from build123d import *

# Parameters (mm, degrees)
F0_R     = 6.604
F0_R_2   = 3.175
F1_DEPTH = 2.54
F2_R     = 10.414
F2_R_2   = 6.604
F2_R_3   = 3.175
F3_DEPTH = 3.81
F4_SIZE  = 3.80999
F6_DEPTH = 6.35


# Not quite as in the source:
# - a fillet or chamfer is up to 0.001 mm smaller than in the source, because OpenCascade refuses the exact size


with BuildPart() as f1:
    # F0 (on Top) → F1 (new body)
    with BuildSketch(Plane.XY):
        Circle(F0_R)
        Circle(F0_R_2, mode=Mode.SUBTRACT)
    extrude(amount=F1_DEPTH)

    # F2 (on face) → F3 (join)
    with BuildSketch(Plane.XY.offset(2.54)):
        Circle(F2_R)
        Circle(F2_R_2, mode=Mode.SUBTRACT)
        Circle(F2_R_2)
        Circle(F2_R_3, mode=Mode.SUBTRACT)
    extrude(amount=F3_DEPTH)

    # F4 (size 3.81 in the source; OpenCascade refuses exactly that, so slightly less here)
    f4_edges = [f1.edges().sort_by_distance(p)[0] for p in [
        (-10.414, 0, 2.54),
    ]]
    chamfer(f4_edges, length=F4_SIZE)

    # F5 (on face) → F6 (join)
    with BuildSketch(Plane.XY.offset(6.35)):
        with BuildLine():
            add(Edge.make_bspline(
                [(0, -10.5673162871), (8.8130461977, -15.2646437839), (9.1515643544, -5.2836581435)],
                knots=[2.3754047296, 2.3754047296, 2.3754047296, 3.9077805776, 3.9077805776, 3.9077805776], degree=2, weights=[1, 0.7205591673, 1]))
            add(Edge.make_bspline(
                [(9.1515643544, -5.2836581435), (17.6260923954, 0), (9.1515643544, 5.2836581435)],
                knots=[5.5169973832, 5.5169973832, 5.5169973832, 7.0493732312, 7.0493732312, 7.0493732312], degree=2, weights=[1, 0.7205591673, 1]))
            add(Edge.make_bspline(
                [(9.1515643544, 5.2836581435), (8.8130461977, 15.2646437839), (0, 10.5673162871)],
                knots=[2.3754047296, 2.3754047296, 2.3754047296, 3.9077805776, 3.9077805776, 3.9077805776], degree=2, weights=[1, 0.7205591673, 1]))
            add(Edge.make_bspline(
                [(0, 10.5673162871), (-8.8130461977, 15.2646437839), (-9.1515643544, 5.2836581435)],
                knots=[5.5169973832, 5.5169973832, 5.5169973832, 7.0493732312, 7.0493732312, 7.0493732312], degree=2, weights=[1, 0.7205591673, 1]))
            add(Edge.make_bspline(
                [(-9.1515643544, 5.2836581435), (-17.6260923954, 0), (-9.1515643544, -5.2836581435)],
                knots=[2.3754047296, 2.3754047296, 2.3754047296, 3.9077805776, 3.9077805776, 3.9077805776], degree=2, weights=[1, 0.7205591673, 1]))
            add(Edge.make_bspline(
                [(-9.1515643544, -5.2836581435), (-8.8130461977, -15.2646437839), (0, -10.5673162871)],
                knots=[5.5169973832, 5.5169973832, 5.5169973832, 7.0493732312, 7.0493732312, 7.0493732312], degree=2, weights=[1, 0.7205591673, 1]))
        make_face()
        Polygon((-6.5991135768, 0), (-3.2995567884, 5.715), (3.2995567884, 5.715), (6.5991135768, 0), (3.2995567884, -5.715), (-3.2995567884, -5.715), align=None, mode=Mode.SUBTRACT)
    extrude(amount=F6_DEPTH)


solid = f1.part
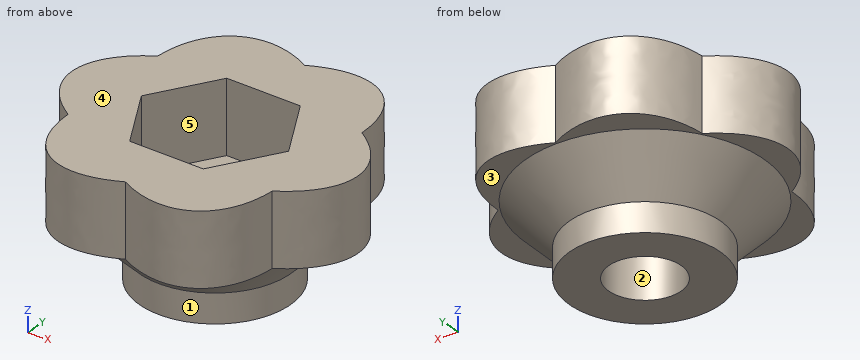
Geometry check sheet. Reference: the model listing, model coordinates, mm. Face numbers are marked on the shaded views. A direction names the side the tool comes from. Give positions to 0.01 mm unless a question says otherwise; leave off trailing zeros. Write each loop counter-clockwise with the first axis right and the second up, starting at its lowest first coordinate (ties: lowest second). Pieces come first, ordered by that corner, then holes. Notation, with made-up numbers: M 1.25,52.25 L 10.25,52.25 A16 ccw 10.25,61.25 Z; hole C 50,76 d6. An arc over 180 degrees is marked long. Answer as CSV lines item,"result". Start each with the question number.
Q1. Release check for a two-part mould opening along Y. For the marked faces 1, 2 and 3 record: pulls with the +Y half, pulls with the -Y half, needs draft (parallel to the pull), parting line crosses it, or undercut.
Q2. Tool access check on the marked faces 4 and 5. Record the directions out of +Z, -Z, +X, -X, +Y, -Y that give a thin tool (end or side, any length) a straight path to the whole face; none if there is none.
Q3. Section check A-A, the plane z = 5.75. Record the cut outline in (x, y) (3 decimals).
Q4. Material ranges on L1, parallel to Z at x = -5.5, y = 0.5; L2, parallel to Z at x = -10.75, y = -0.5; L3, parallel to Y at x = 0, z = 4.25 (3 decimals), recorded low to high.
Q5. Go/stop test with flat-tipped pins: pin 1 (3 mm diameter, centred on x = 8.5, y = 3.5, fed in from -Z); pin 2 (1.9 mm diameter, centred on x = -0.5, z = 10.5, fed in from +Y); pin 3 (1.5 mm diameter, centred on x = 2.5, z = 3, fed in from +Y). Record where each tip stops, or that it passes through.
Geometry says:
1,face 1,"parting line crosses it"
1,face 2,"undercut"
1,face 3,"needs draft"
2,face 4,"+Z, +X, -X, +Y, -Y"
2,face 5,"+Z"
3,outline,"C 0,0 d19.628; hole C 0,0 d6.35"
4,L1,"0 to 6.35"
4,L2,"6.35 to 12.7"
4,L3,"-8.314 to -3.175, 3.175 to 8.314"
5,pin 1,"z = 3.63"
5,pin 2,"y = 11.21"
5,pin 3,"y = 7.44"
